Design review of the part built by this model. Coordinates are the model's own, in mm. A direction names the side the tool comes from. Round coordinates to 2 decimals unless told otherwise and drop trailing zeros. Order: outer loops, then holes, each group sorted by start corner. A loop starts at its lowest first (then second) coordinate and runs counter-clockwise, first axis right, second up. Notation, with made-up numbers: (68.5, 82.5) - (121.5, 82.5) arc R26 cw to (121.5, 109.5) - close; hole circle Ø9 at (70, 47). An arc over 180 degrees is marked (long way). Write item = value, one per line.
from build123d import *

# Parameters (mm, degrees)
F0_R     = 19.05
F1_DEPTH = 63.5
F2_DEPTH = 63.5
F4_DEPTH = 4.7752
F5_DEPTH = 25.4
F6_DEPTH = 15.875
F7_R     = 6.1341
F8_DEPTH = 25.4


with BuildPart() as f1:
    # F0 (on Front) → F1 (new body)
    with BuildSketch(Plane.XZ):
        with BuildLine():
            Line((79.502, 28.575), (0, 28.575))
            ThreePointArc((0, 28.575), (-19.345366451, -21.0306305629), (28.4756083945, 2.38125))
            ThreePointArc((28.4756083945, 2.38125), (30.9572676717, 9.6234554837), (37.9674778593, 12.7))
            Line((37.9674778593, 12.7), (79.502, 12.7))
            Line((79.502, 12.7), (79.502, 28.575))
        make_face()
        Circle(F0_R, mode=Mode.SUBTRACT)
    extrude(amount=F1_DEPTH)

    # F0 (on Front) → F2 (join)
    with BuildSketch(Plane.XZ):
        with BuildLine():
            Line((79.502, 28.575), (0, 28.575))
            ThreePointArc((0, 28.575), (-19.345366451, -21.0306305629), (28.4756083945, 2.38125))
            ThreePointArc((28.4756083945, 2.38125), (30.9572676717, 9.6234554837), (37.9674778593, 12.7))
            Line((37.9674778593, 12.7), (79.502, 12.7))
            Line((79.502, 12.7), (79.502, 28.575))
        make_face()
        Circle(F0_R, mode=Mode.SUBTRACT)
    extrude(amount=F2_DEPTH)

    # F3 (on face) → F4 (join)
    with BuildSketch(Plane.XY.offset(28.575)):
        with BuildLine():
            ThreePointArc((86.5250683207, -42.3314229366), (83.1698282884, -43.9088254222), (79.502, -44.45))
            Line((79.502, -44.45), (79.502, -46.992751468))
            Line((79.502, -46.992751468), (86.5250683207, -42.3314229366))
        make_face()
        with BuildLine():
            Line((86.5250683207, -21.1685770634), (79.502, -16.507248532))
            Line((79.502, -16.507248532), (79.502, -19.05))
            ThreePointArc((79.502, -19.05), (83.1698282884, -19.5911745778), (86.5250683207, -21.1685770634))
        make_face()
        with BuildLine():
            ThreePointArc((86.5250683207, -21.1685770634), (83.1698282884, -19.5911745778), (79.502, -19.05))
            Line((79.502, -19.05), (79.502, -44.45))
            ThreePointArc((79.502, -44.45), (83.1698282884, -43.9088254222), (86.5250683207, -42.3314229366))
            ThreePointArc((86.5250683207, -42.3314229366), (92.202, -31.75), (86.5250683207, -21.1685770634))
        make_face()
        with BuildLine():
            ThreePointArc((57.8230683207, -2.1185770634), (54.467828274, -0.5411745735), (50.7999999699, 0))
            ThreePointArc((50.7999999699, 0), (41.8197438683, -3.7197438896), (38.1, -12.7))
            Line((38.1, -12.7), (38.1, -50.8))
            ThreePointArc((38.1, -50.8), (41.8197438789, -59.7802561211), (50.8, -63.5))
            ThreePointArc((50.8, -63.5), (54.4678282884, -62.9588254222), (57.8230683207, -61.3814229366))
            Line((57.8230683207, -61.3814229366), (79.502, -46.992751468))
            Line((79.502, -46.992751468), (79.502, -44.45))
            Line((79.502, -44.45), (79.502, -19.05))
            Line((79.502, -19.05), (79.502, -16.507248532))
            Line((79.502, -16.507248532), (57.8230683207, -2.1185770634))
        make_face()
    extrude(amount=F4_DEPTH)

    # F5 (cut): faces of the model
    f5_faces = [f1.faces().sort_by_distance(p)[0] for p in [
        (71.0984865621, -5.4680526569, 28.575),
        (71.0984865621, -58.0319473431, 28.575),
    ]]
    extrude(f5_faces, amount=-F5_DEPTH, mode=Mode.SUBTRACT)

    # F6 (add): a face of the model
    f6_faces = [f1.faces().sort_by_distance(p)[0] for p in [
        (84.7235761058, -31.75, 28.575),
    ]]
    extrude(f6_faces, amount=F6_DEPTH)

    # F7 (on face) → F8 (cut)
    with BuildSketch(Plane.XY.offset(33.3502)):
        with Locations((50.8, -12.7)):
            Circle(F7_R)
        with Locations((79.502, -31.75)):
            Circle(F7_R)
        with Locations((50.8, -50.8)):
            Circle(F7_R)
    extrude(amount=-F8_DEPTH, mode=Mode.SUBTRACT)


solid = f1.part
Item 1: Insertion check: P1, Ø15, axis at x = 23.5, y = -31, coming from the +Z side (3 decimals); P2, Ø16, axis at x = 50.8, y = -50.8, coming from the -Z side; P3, Ø7.5, axis at x = 50.8, y = -12.7, coming from the +Z side; P4, Ø12, axis at y = -28.5, z = 2, coming from the +X side (3 decimals). Each pin has a flat end and moves straight along its axis. Give the tip position at first contact, or say it passes through.
Data:
P1 = 28.575
P2 = 12.7
P3 = through
P4 = 29.755
Item 2: Take a section at C-C, the plane x = -10. State the section outline as (y, z) points.
Data:
outline = (-63.5, -26.77) - (0, -26.77) - (0, -16.21) - (-63.5, -16.21) - close; (-63.5, 16.21) - (0, 16.21) - (0, 26.77) - (-63.5, 26.77) - close
Item 3: The part is to be moulded in two halves that separate along Y. For faces 4 (the face through (19, -63.5, 7)), 5 (the face through (56.65, -10.86, 23.17)), 6 (the face through (30.88, -31.31, 9.54)), say which applies: +Y half, -Y half, draft (parallel to the pull), parting line (faces both ways), or undercut.
Data:
face_4 = -Y half
face_5 = undercut
face_6 = draft
Item 4: For faces 1 (the face through (59, -31, 33.35)), 2 (the face through (59, -31, 12.7)), 3 (the face through (38.1, -31, 31)), list the 3-axis set-ups (+Z, -Z, +X, -X, +Y, -Y) from which the entire face can be reached by the end or side of a thin tool; tool diameter is ignored.
Data:
face_1 = +Z, +X, -X, +Y, -Y
face_2 = -Z, +X, +Y, -Y
face_3 = +Z, -X, +Y, -Y
Item 5: Take a section at A-A, the plane y = -11. State the section outline as (x, z) points (3 decimals).
Data:
outline = (0, 28.575) arc R28.575 ccw (long way) to (28.476, 2.381) arc R9.525 cw to (37.967, 12.7) - (44.906, 12.7) - (44.906, 33.35) - (38.214, 33.35) - (38.214, 28.575) - close; (56.694, 12.7) - (71.204, 12.7) - (71.204, 33.35) - (56.694, 33.35) - close; hole circle Ø38.1 at (0, 0)
Item 6: For line 1 along X through (y, z) = (-42.5, -0.5); line 2 along Z through (x, y) = (64, -42.5); line 3 along Z through (x, y) = (10, -43.5) (3 decimals), list the stretches that pass through material, from the lowest coordinate up. Write a range as [from, to].
Data:
line_1 = [-28.57, -19.04], [19.04, 28.57]
line_2 = [12.7, 33.35]
line_3 = [-26.768, -16.214], [16.214, 28.575]
Item 7: Take a section at D-D, the plane y = -31.75. State the section outline as (x, z) points (3 decimals).
Data:
outline = (0, 28.575) arc R28.575 ccw (long way) to (28.476, 2.381) arc R9.525 cw to (37.967, 12.7) - (73.368, 12.7) - (73.368, 33.35) - (38.1, 33.35) - (38.1, 28.575) - close; (85.636, 12.7) - (92.202, 12.7) - (92.202, 33.35) - (85.636, 33.35) - close; hole circle Ø38.1 at (0, 0)
Item 8: Take a section at B-B, the plane z = 0. State the section outline as (x, y) points (3 decimals).
Data:
outline = (-28.575, -63.5) - (-19.05, -63.5) - (-19.05, 0) - (-28.575, 0) - close; (19.05, -63.5) - (28.575, -63.5) - (28.575, 0) - (19.05, 0) - close
